```python
from build123d import *

# Parameters (mm, degrees)
F1_DEPTH  = 35
F5_DEPTH  = 13
F7_DEPTH  = 13
F9_D      = 6.6
F12_DEPTH = 15
F14_D     = 8.6
F17_D     = 6
F17_DEPTH = 10
F17_TIP   = 1.8025818571
F19_D     = 6
F19_DEPTH = 10
F19_TIP   = 1.8025818571


with BuildPart() as f1:
    # F0 (on Front) → F1 (new body, symmetric)
    with BuildSketch(Plane.XZ):
        Polygon((50, 23.3153829077), (0, 0), (50, 0), align=None)
    extrude(amount=F1_DEPTH, both=True)

    # F4 (on face) → F5 (join)
    with BuildSketch(Plane.XZ.offset(35)):
        Polygon((0, 5.5168895948), (0, 0), (50, 23.3153829077), (50, 28.8322725026), align=None)
    extrude(amount=-F5_DEPTH)

    # F6 (on face) → F7 (join)
    with BuildSketch(Plane(origin=(0, 35, 0), x_dir=(-1, 0, 0), z_dir=(0, 1, 0))):
        Polygon((-50, 28.832308948), (-50, 23.3153829077), (0, 0), (0, 5.5180899799), align=None)
    extrude(amount=-F7_DEPTH)

    # F9 (through all)
    with Locations(Plane(origin=(-2.1134832591, 0, 4.5326057501), x_dir=(0.9063158679, 0, 0.4226009319), z_dir=(-0.4226009319, 0, 0.9063158679))):
        with Locations((26.3319499681, 28), (26.3319499681, -28)):
            Hole(F9_D / 2)

    # F11 (on offset) → F12 (cut)
    with BuildSketch(Plane(origin=(2.1130913087, 0, -4.5315389352), x_dir=(0.906307787, 0, 0.4226182617), z_dir=(0.4226182617, 0, -0.906307787))):
        Polygon((20.2118023361, -28), (23.2717587628, -33.3), (29.3916716162, -33.3), (32.4516280429, -28), (29.3916716162, -22.7), (23.2717587628, -22.7), align=None)
        Polygon((20.2118023361, 28), (23.2717587628, 22.7), (29.3916716162, 22.7), (32.4516280429, 28), (29.3916716162, 33.3), (23.2717587628, 33.3), align=None)
    extrude(amount=F12_DEPTH, mode=Mode.SUBTRACT)

    # F14 (through all)
    with Locations(Plane.XZ.offset(35)):
        with Locations((43, 9)):
            Hole(F14_D / 2)

    # F17
    with Locations(Plane.XZ.offset(35)):
        with Locations((15, 5)):
            Hole(F17_D / 2, depth=F17_DEPTH)
            with Locations((0, 0, -(F17_DEPTH + F17_TIP / 2))):  # 118° drill point
                Cone(0, F17_D / 2, F17_TIP, mode=Mode.SUBTRACT)

    # F19
    with Locations(Plane(origin=(0, 35, 0), x_dir=(-1, 0, 0), z_dir=(0, 1, 0))):
        with Locations((-15, 5)):
            Hole(F19_D / 2, depth=F19_DEPTH)
            with Locations((0, 0, -(F19_DEPTH + F19_TIP / 2))):  # 118° drill point
                Cone(0, F19_D / 2, F19_TIP, mode=Mode.SUBTRACT)


solid = f1.part
```
Read the model definition and answer for the solid it produces. Units are mm, in the model's axes. A direction names the side the tool comes from. Round coordinates to 2 decimals unless told otherwise and drop trailing zeros. Write each loop counter-clockwise with the first axis right and the second up, starting at its lowest first coordinate (ties: lowest second). Pieces come first, ordered by that corner, then holes. Notation, with made-up numbers: (-34.5, 47.5) - (-6.5, 47.5) arc R37 ccw to (-6.5, 84.5) - close; hole circle Ø2 at (23.5, -8). An arc over 180 degrees is marked (long way). One line per item, written item: value.
Q1. Straight lines are drawn through the part: line 1 (Y direction, x = 26.5, z = 4); line 2 (Y direction, x = 25.5, z = 9.75); line 3 (X direction, y = -1, z = 11.5). For each, find the intervals that lie inside material, in ascending order. Write a range as from..to.
The answers:
line 1: y = -35..-33.3, -22.7..22.7, 33.3..35
line 2: y = -35..-31.18, -24.82..24.82, 31.18..35
line 3: x = 24.66..39.5, 46.5..50
Q2. Find section A-A (x = 41). Determine the outline of the cut face in (y, z), and give its area (3 significant figures).
The answers:
outline: (-35, 0) - (35, 0) - (35, 5.19) - (-35, 5.19) - close; (-35, 12.81) - (35, 12.81) - (35, 24.64) - (22, 24.64) - (22, 19.12) - (-22, 19.12) - (-22, 24.64) - (-35, 24.64) - close
area: 949 mm2
Q3. Find section C-C (x = 10.5). Determine the outline of the cut face in (y, z), and give its area (3 significant figures).
The answers:
outline: (-35, 0) - (35, 0) - (35, 10.41) - (22, 10.41) - (22, 4.9) - (-22, 4.9) - (-22, 10.41) - (-35, 10.41) - close
area: 486 mm2
Q4. Which of the six approach directions +Z, -Z, +X, -X, +Y, -Y give full straight-line access (tool end or side, diameter ignored) to faces 4 (the flat face through (32.23, 30.69, 4)), 5 (the flat face through (25, -22, 13)), 6 (the flat face through (0, -29, 3)), 7 (the flat face through (28.365, -30.43, 7.71)), 8 (the flat face through (50, 0, 15))?
The answers:
face 4: -Z
face 5: +Z, -X
face 6: +Z, -Z, -X, +Y, -Y
face 7: none
face 8: +Z, -Z, +X, +Y, -Y
Q5. Each of these flat-tipped pins is pushed along its axis until it touches: P1, Ø1, axis at y = -12, z = 7.5, coming from the -X side; P2, Ø5, axis at x = 15, z = 5, coming from the -Y side; P3, Ø8, axis at y = -7.5, z = 21.5, coming from the -X side. Where does it stop, or does it pass through?
The answers:
P1: stops at x = 15.01
P2: stops at y = -24.7
P3: stops at x = 37.53
Q6. For a pull along Z with two mould halves and no side action, classify faces 1 (the flat face through (25.35, -28.591, 17.338)), 2 (the cylindrical face through (17.4, -29.9, 3.2)), 3 (the flat face through (0, 29, 3)) as pulls with the +Z half, pulls with the -Z half, needs draft (parallel to the pull), parting line crosses it, or undercut.
The answers:
face 1: pulls with the +Z half
face 2: undercut
face 3: needs draft
Q7. Find section B-B (y = -18.5). Determine the outline of the cut face in (x, z), and give its area (3 significant figures).
The answers:
outline: (0, 0) - (50, 0) - (50, 23.32) - close; hole circle Ø8.6 at (43, 9)
area: 525 mm2
